Build history of the part. All positions in model axes, mm. Face numbers are marked on the shaded views. A direction names the side the tool comes from. Round coordinates to 2 decimals unless told otherwise and drop trailing zeros. Order: outer loops, then holes, each group sorted by start corner. A loop starts at its lowest first (then second) coordinate and runs counter-clockwise, first axis right, second up. Notation, with made-up numbers: (45, 39.25) -> (69, 39.25) arc R19 cw to (69, 76.25) -> close; hole circle Ø9 at (39.5, 3.25). An arc over 180 degrees is marked (long way). Use a Markdown table: item, result. Add a question column.
Item 1: Slice it at D-D, the plane y = 25.5. Give the cut face in (x, z).
Item 2: Two-plate mould, pull along X, no slides. Class the marked faces 1, 2 and 3: released by +X, released by -X, zero draft, split by the parting line, or undercut.
Item 3: Slice it at C-C, the plane x = 0. Give the cut face in (y, z).
Item 4: Slice it at A-A, the plane x = 12.75. Give the cut face in (y, z).
Item 5: 3-axis set-ups, long thin cutter, end or side, ignore diameter. For the marked faces 4, 5, 6, 7 and 8: which of +Z, -Z, +X, -X, +Y, -Y reach the whole face in a straight line?
Item 6: Pin check, flat tips, straight feed: pin 1 (2.5 mm diameter, centred on x = 0, z = 0, fed in from -Y); pin 2 (15.5 mm diameter, centred on x = -5.5, y = 24, fed in from +Z); pin 3 (3 mm diameter, centred on x = 0.5, z = 23, fed in from +Y); pin 4 (10 mm diameter, centred on y = 11.5, z = 25.5, fed in from -X). Stop position of each tip, or through.
Item 7: Probe L1, parallel to X at y = 32, z = 0; L2, parallel to Z at x = 3.5, y = 17.5; L3, parallel to Z at x = -4.5, y = 8.5. List the from-to ranges inside material, lowest first.
Item 8: Slice it at B-B, the plane z = 0. Give the cut face in (x, y), plus the area to 3 significant figures.
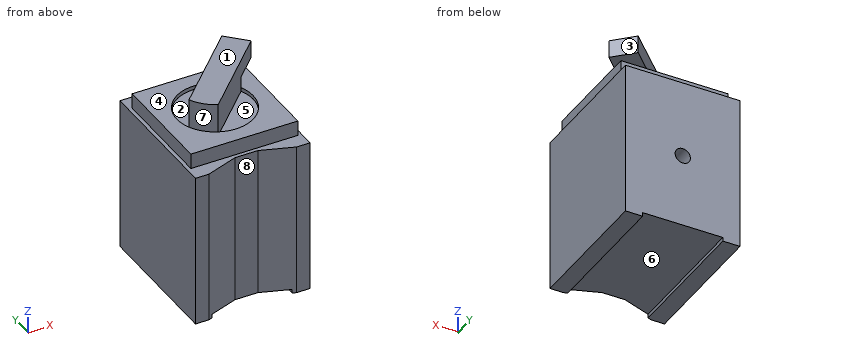
from build123d import *

# Parameters (mm, degrees)
SKETCH_1_W          = 30
SKETCH_1_H          = 40.5
EXTRUDE_1_DEPTH     = 36
SKETCH_2_W          = 28
SKETCH_2_H          = 28
EXTRUDE_2_DEPTH     = 4
SKETCH_3_R          = 10
CUT_EXTRUDE_1_DEPTH = 1
EXTRUDE_START       = 4
EXTRUDE_3_DEPTH     = 4
EXTRUDE_START_2     = 4.6
EXTRUDE_4_DEPTH     = 4.6
SKETCH_7_W          = 21
SKETCH_7_H          = 1
CUT_EXTRUDE_2_DEPTH = 51.352979058
CUT_EXTRUDE_3_DEPTH = 57.224994442
SKETCH_9_R          = 2
CUT_EXTRUDE_4_DEPTH = 6.5


with BuildPart() as part:
    # 草图1 → 凸台-拉伸1 (new body)
    with BuildSketch(Plane(origin=(0, 0, 0), x_dir=(1, 0, 0), z_dir=(0, 1, 0))):
        Rectangle(SKETCH_1_W, SKETCH_1_H)
    extrude(amount=EXTRUDE_1_DEPTH)

    # 草图2 → 凸台-拉伸2 (add)
    with BuildSketch(Plane.XY.offset(20.25)):
        with Locations((0, 18)):
            Rectangle(SKETCH_2_W, SKETCH_2_H)
    extrude(amount=EXTRUDE_2_DEPTH)

    # 草图3 → 切除-拉伸1 (cut)
    with BuildSketch(Plane.XY.offset(24.25)):
        with Locations((0, 18)):
            Circle(SKETCH_3_R)
    extrude(amount=-CUT_EXTRUDE_1_DEPTH, mode=Mode.SUBTRACT)

    # 草图5 → 凸台-拉伸3 (add)
    with BuildSketch(Plane.XY.offset(23.25).offset(EXTRUDE_START)):
        with BuildLine():
            Line((4.148946916, 27.098694384), (-9.098694384, 13.851053084))
            ThreePointArc((-9.098694384, 13.851053084), (-7.071067812, 10.928932188), (-4.148946916, 8.901305616))
            Line((-4.148946916, 8.901305616), (9.098694384, 22.148946916))
            ThreePointArc((9.098694384, 22.148946916), (7.071067812, 25.071067812), (4.148946916, 27.098694384))
        make_face()
    extrude(amount=-EXTRUDE_3_DEPTH)

    # 草图6 → 凸台-拉伸4 (add)
    with BuildSketch(Plane.XY.offset(27.25).offset(EXTRUDE_START_2)):
        with BuildLine():
            Line((-9.098694384, 13.851053084), (9.993188708, 32.942936176))
            Line((9.993188708, 32.942936176), (14.942936176, 27.993188708))
            Line((14.942936176, 27.993188708), (-4.148946916, 8.901305616))
            ThreePointArc((-4.148946916, 8.901305616), (-7.071067812, 10.928932188), (-9.098694384, 13.851053084))
        make_face()
    extrude(amount=-EXTRUDE_4_DEPTH)

    # 草图7 → 切除-拉伸2 (cut, through all)
    with BuildSketch(Plane(origin=(0, 36, 0), x_dir=(1, 0, 0), z_dir=(0, 1, 0))):
        with Locations((0, 19.75)):
            Rectangle(SKETCH_7_W, SKETCH_7_H)
    extrude(amount=-CUT_EXTRUDE_2_DEPTH, mode=Mode.SUBTRACT)

    # 草图8 → 切除-拉伸3 (cut, through all)
    with BuildSketch(Plane.XY.offset(20.25)):
        Polygon((-11.5, 0), (-3, 3), (3, 3), (11.5, 0), align=None)
    extrude(amount=-CUT_EXTRUDE_3_DEPTH, mode=Mode.SUBTRACT)

    # 草图9 → 切除-拉伸4 (cut)
    with BuildSketch(Plane(origin=(0, 36, 0), x_dir=(1, 0, 0), z_dir=(0, 1, 0))):
        with Locations(Location((0, 0, 0), (0, 0, 270))):
            Circle(SKETCH_9_R)
    extrude(amount=-CUT_EXTRUDE_4_DEPTH, mode=Mode.SUBTRACT)


solid = part.part
Check sheet entries:
| question | item | result |
|---|---|---|
| 1 | outline | (-15, -20.25) -> (-10.5, -20.25) -> (-10.5, -19.25) -> (10.5, -19.25) -> (10.5, -20.25) -> (15, -20.25) -> (15, 20.25) -> (14, 20.25) -> (14, 24.25) -> (6.61, 24.25) -> (6.61, 27.25) -> (12.45, 27.25) -> (12.45, 31.85) -> (2.55, 31.85) -> (2.55, 23.25) -> (-6.61, 23.25) -> (-6.61, 24.25) -> (-14, 24.25) -> (-14, 20.25) -> (-15, 20.25) -> close |
| 2 | face 1 | zero draft |
| 2 | face 2 | undercut |
| 2 | face 3 | released by +X |
| 3 | outline | (3, -19.25) -> (36, -19.25) -> (36, -2) -> (29.5, -2) -> (29.5, 2) -> (36, 2) -> (36, 20.25) -> (32, 20.25) -> (32, 24.25) -> (28, 24.25) -> (28, 23.25) -> (22.95, 23.25) -> (22.95, 31.85) -> (13.05, 31.85) -> (13.05, 23.25) -> (8, 23.25) -> (8, 24.25) -> (4, 24.25) -> (4, 20.25) -> (3, 20.25) -> close |
| 4 | outline | (0, -20.25) -> (36, -20.25) -> (36, 20.25) -> (32, 20.25) -> (32, 24.25) -> (4, 24.25) -> (4, 20.25) -> (0, 20.25) -> close; (25.8, 27.25) -> (30.19, 27.25) -> (30.19, 31.85) -> (25.8, 31.85) -> close |
| 5 | face 4 | none |
| 5 | face 5 | +Z |
| 5 | face 6 | -Z, +Y, -Y |
| 5 | face 7 | +Z, -X, -Y |
| 5 | face 8 | +Z, -Z, -Y |
| 6 | pin 1 | y = 3 |
| 6 | pin 2 | z = 31.85 |
| 6 | pin 3 | y = 32 |
| 6 | pin 4 | x = -14 |
| 7 | L1 | -15 to -2, 2 to 15 |
| 7 | L2 | -19.25 to 31.85 |
| 7 | L3 | -19.25 to 24.25 |
| 8 | outline | (-15, 0) -> (-11.5, 0) -> (-3, 3) -> (3, 3) -> (11.5, 0) -> (15, 0) -> (15, 36) -> (2, 36) -> (2, 29.5) -> (-2, 29.5) -> (-2, 36) -> (-15, 36) -> close |
| 8 | area | 1,010 mm2 |
